```python
from build123d import *

# Parameters (mm, degrees)
SKETCH001_R       = 0.45
PAD001_DEPTH      = 12.25
PAD001_DEPTH_BACK = 3.5
SKETCH_R          = 7.1
PAD_DEPTH         = 24.5
FILLET_R          = 0.5


with BuildPart() as pad001:
    # Sketch001 → Pad001 (new body, two sides)
    with BuildSketch(Plane.XY.offset(0.5)) as pad001_sk:
        Circle(SKETCH001_R)
        with Locations((10, 0)):
            Circle(SKETCH001_R)
    extrude(amount=PAD001_DEPTH)
    extrude(pad001_sk.sketch, amount=-PAD001_DEPTH_BACK)


with BuildPart() as obj1:
    # Sketch → Pad (new body)
    with BuildSketch(Plane.XY.offset(0.1)):
        with Locations((5, 0)):
            Circle(SKETCH_R)
    extrude(amount=PAD_DEPTH)

    # Fillet
    fillet_edges = [obj1.edges().sort_by_distance(p)[0] for p in [
        (-2.1, 0, 0.1),
        (-2.1, 0, 24.6),
    ]]
    fillet(fillet_edges, radius=FILLET_R)

    add(pad001.part)


solid = obj1.part
```
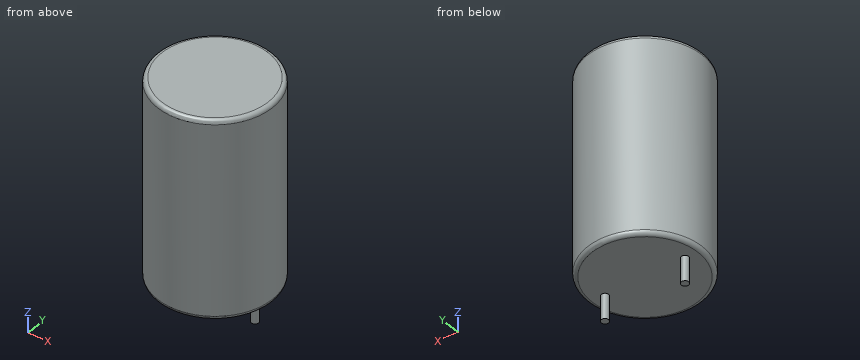
Geometry check sheet. Reference: the model listing, model coordinates, mm. Coordinates: 2 decimals unless noted, no trailing zeros. Order: outer loops, then holes, each group sorted by start corner. A loop starts at its lowest first (then second) coordinate and runs counter-clockwise, first axis right, second up. Notation, with made-up numbers: (76.5, 86.25) - (99.5, 86.25) arc R18 ccw to (99.5, 102.25) - close; hole circle Ø3 at (27.25, -8.75). An arc over 180 degrees is marked (long way). Use one line per item in the form item = value.
1. Section check B-B (z = 14.5). Record the boundary of the cut face in (x, y), then the cut area to 3 significant figures.
Here are the results:
outline = circle Ø14.2 at (5, 0)
area = 158 mm²
2. Section check A-A (x = 5). Record the boundary of the cut face in (y, z).
Here are the results:
outline = (-7.1, 0.6) arc R0.5 ccw to (-6.6, 0.1) - (6.6, 0.1) arc R0.5 ccw to (7.1, 0.6) - (7.1, 24.1) arc R0.5 ccw to (6.6, 24.6) - (-6.6, 24.6) arc R0.5 ccw to (-7.1, 24.1) - close
3. Scan lines: line 1 (Z direction, x = 2.25, y = -5); line 2 (X direction, y = -0.25, z = 21); line 3 (Y direction, x = 4.75, z = 10.25). Record each from-to range of solid material in increasing order.
Here are the results:
line_1 = 0.1 to 24.6
line_2 = -2.1 to 12.1
line_3 = -7.1 to 7.1
4. Gauge pin test, flat ends, axial feed: pin 1 (1 mm diameter, centred on x = 5, y = -3, fed in from -Z); pin 2 (2 mm diameter, centred on x = 7, z = 12.5, fed in from -Y); pin 3 (1.5 mm diameter, centred on y = 5, z = 1.5, fed in from -X); pin 4 (5 mm diameter, centred on y = -2.5, z = 18.5, fed in from +X). Record the tip position at first contact, or that the pin passes through.
Here are the results:
pin_1 = 0.1
pin_2 = -7.03
pin_3 = -0.69
pin_4 = 12.1
